from build123d import *

# Parameters (mm, degrees)
ESQUISSE1_W                                       = 50
ESQUISSE1_H                                       = 60
ESQUISSE1_R                                       = 14.5
BOSS_EXTRU_1_DEPTH                                = 10
ESQUISSE2_R                                       = 21.3
BOSS_EXTRU_2_DEPTH                                = 65.3
BOSS_EXTRU_3_START                                = -25
BOSS_EXTRU_3_DEPTH                                = 25
ENL_V_START                                       = 22
ENL_V_MAT_EXTRU_1_DEPTH                           = 22
CHAMBRAGE_POUR_VIS_SIX_PANS_CREUX_M41_D           = 4.5
CHAMBRAGE_POUR_VIS_SIX_PANS_CREUX_M41_CBORE_D     = 8
CHAMBRAGE_POUR_VIS_SIX_PANS_CREUX_M41_CBORE_DEPTH = 4.4
CHAMBRAGE_POUR_VIS_SIX_PANS_CREUX_M42_D           = 4.8
CHAMBRAGE_POUR_VIS_SIX_PANS_CREUX_M42_CBORE_D     = 8
CHAMBRAGE_POUR_VIS_SIX_PANS_CREUX_M42_CBORE_DEPTH = 4.4
BOSS_EXTRU_4_DEPTH                                = 30
CONG_1_R                                          = 4
CONG_2_R                                          = 4


with BuildPart() as part:
    # Esquisse1 → Boss.-Extru.1 (new body)
    with BuildSketch(Plane(origin=(0, 0, 0), x_dir=(1, 0, 0), z_dir=(0, 1, 0))):
        with Locations((25, 30)):
            Rectangle(ESQUISSE1_W, ESQUISSE1_H)
        with Locations(Location((25, 30, 0), (0, 0, 270))):
            Circle(ESQUISSE1_R, mode=Mode.SUBTRACT)
    extrude(amount=BOSS_EXTRU_1_DEPTH)

    # Esquisse2 → Boss.-Extru.2 (add)
    with BuildSketch(Plane(origin=(0, 10, 0), x_dir=(1, 0, 0), z_dir=(0, 1, 0))):
        with BuildLine():
            ThreePointArc((50, 41.456439237), (25, 57.5), (0, 41.456439237))
            Line((0, 41.456439237), (0, 18.543560763))
            ThreePointArc((0, 18.543560763), (25, 2.5), (50, 18.543560763))
            Line((50, 18.543560763), (50, 41.456439237))
        make_face()
        with Locations(Location((25, 30, 0), (0, 0, 270))):
            Circle(ESQUISSE2_R, mode=Mode.SUBTRACT)
    extrude(amount=BOSS_EXTRU_2_DEPTH)

    # Esquisse3 → Boss.-Extru.3 (add)
    with BuildSketch(Plane(origin=(0, 75.3, 0), x_dir=(1, 0, 0), z_dir=(0, 1, 0)).offset(BOSS_EXTRU_3_START)):
        with BuildLine():
            ThreePointArc((50, 18.543560763), (49.08967559, 16.735855475), (48.048861143, 15))
            Line((48.048861143, 15), (62.5, 15))
            Line((62.5, 15), (62.5, 45))
            Line((62.5, 45), (48.048861143, 45))
            ThreePointArc((48.048861143, 45), (49.08967559, 43.264144525), (50, 41.456439237))
            ThreePointArc((50, 41.456439237), (51.867731575, 35.8630197), (52.5, 30))
            ThreePointArc((52.5, 30), (51.867731575, 24.1369803), (50, 18.543560763))
        make_face()
        with BuildLine():
            Line((50, 41.456439237), (50, 18.543560763))
            ThreePointArc((50, 18.543560763), (51.867731575, 24.1369803), (52.5, 30))
            ThreePointArc((52.5, 30), (51.867731575, 35.8630197), (50, 41.456439237))
        make_face()
    extrude(amount=BOSS_EXTRU_3_DEPTH)

    # Esquisse4 → Enlèv. mat.-Extru.1 (cut)
    with BuildSketch(Plane(origin=(0, 75.3, -75.3), x_dir=(1, 0, 0), z_dir=(0, -1, 0)).offset(ENL_V_START)):
        with BuildLine():
            ThreePointArc((46.3, 45.3), (45.777219327, 40.609887311), (44.234539246, 36.15))
            Line((44.234539246, 36.15), (60, 36.15))
            Line((60, 36.15), (60, 54.45))
            Line((60, 54.45), (44.234539246, 54.45))
            ThreePointArc((44.234539246, 54.45), (45.777219327, 49.990112689), (46.3, 45.3))
        make_face()
    extrude(amount=-ENL_V_MAT_EXTRU_1_DEPTH, mode=Mode.SUBTRACT)

    # Chambrage pour vis à six pans creux M41 (through all)
    with Locations(Plane(origin=(5, 10, -55), x_dir=(0, 0, 1), z_dir=(0, 1, 0))):
        with Locations((0, 0), (0, 40), (50, 40), (50, 0)):
            CounterBoreHole(CHAMBRAGE_POUR_VIS_SIX_PANS_CREUX_M41_D / 2, CHAMBRAGE_POUR_VIS_SIX_PANS_CREUX_M41_CBORE_D / 2, CHAMBRAGE_POUR_VIS_SIX_PANS_CREUX_M41_CBORE_DEPTH)

    # Chambrage pour vis à six pans creux M42 (through all)
    with Locations(Plane(origin=(25, 0, -12.5), x_dir=(0, 0, -1), z_dir=(0, -1, 0))):
        with Locations((0, 0), (17.5, 17.5), (35, 0), (17.5, -17.5)):
            CounterBoreHole(CHAMBRAGE_POUR_VIS_SIX_PANS_CREUX_M42_D / 2, CHAMBRAGE_POUR_VIS_SIX_PANS_CREUX_M42_CBORE_D / 2, CHAMBRAGE_POUR_VIS_SIX_PANS_CREUX_M42_CBORE_DEPTH)

    # Esquisse11 → Boss.-Extru.4 (add)
    with BuildSketch(Plane.XY.offset(-15)):
        Polygon((48.048861143, 50.3), (48.048861143, 15.134837214), (62.5, 50.3), align=None)
    extrude(amount=-BOSS_EXTRU_4_DEPTH)

    # Congé1
    cong_1_edges = [part.edges().sort_by_distance(p)[0] for p in [
        (0, 5, -60),
        (50, 5, -60),
        (50, 5, 0),
        (0, 5, 0),
    ]]
    fillet(cong_1_edges, radius=CONG_1_R)

    # Congé2
    # the kernel refuses this fillet: 4 mm, written as the material it takes off along each edge
    with BuildSketch(Plane(origin=(58.5, 51.089853485, -41), x_dir=(1, 0, 0), z_dir=(0, 0, -1))) as cong_2_piece_1_section:
        Polygon((0, 0), (CONG_2_R, 0), (CONG_2_R, CONG_2_R * 0.197463371222), (CONG_2_R * 0.924943038794, CONG_2_R * 0.38010574185), align=None)
    cong_2_piece_1 = extrude(amount=CONG_2_R, mode=Mode.PRIVATE)
    cong_2_piece_1 = cong_2_piece_1 - Plane(origin=(58.5, 51.089853485, -41), x_dir=(-0.9810563283506197, 0.19372268995448388, 0), z_dir=(0, 0, -1)) * Sphere(CONG_2_R, mode=Mode.PRIVATE)
    add(cong_2_piece_1, mode=Mode.SUBTRACT)
    with BuildSketch(Plane(origin=(58.5, 51.089853485, -19), x_dir=(1, 0, 0), z_dir=(0, 0, 1))) as cong_2_piece_2_section:
        Polygon((0, 0), (CONG_2_R, 0), (CONG_2_R, -CONG_2_R * 0.197463371222), (CONG_2_R * 0.924943038794, -CONG_2_R * 0.38010574185), align=None)
    cong_2_piece_2 = extrude(amount=CONG_2_R, mode=Mode.PRIVATE)
    cong_2_piece_2 = cong_2_piece_2 - Plane(origin=(58.5, 51.089853485, -19), x_dir=(-0.9810563283506197, 0.19372268995448388, 0), z_dir=(0, 0, 1)) * Sphere(CONG_2_R, mode=Mode.PRIVATE)
    add(cong_2_piece_2, mode=Mode.SUBTRACT)
    with BuildSketch(Plane(origin=(62.5, 51.089853485, -45), x_dir=(-1, 0, 0), z_dir=(0, 1, 0))) as cong_2_piece_3:
        with BuildLine():
            CenterArc((CONG_2_R, CONG_2_R), CONG_2_R, 180, 90)
            Line((0, CONG_2_R), (0, 0))
            Line((0, 0), (CONG_2_R, 0))
        make_face()
    extrude(amount=34.210146515, mode=Mode.SUBTRACT)
    with BuildSketch(Plane(origin=(62.5, 50.3, -19), x_dir=(-0.3801057418499003, -0.9249430387935988, 0), z_dir=(0, 0, -1))) as cong_2_piece_4:
        with BuildLine():
            CenterArc((CONG_2_R * 0.197463371222, CONG_2_R), CONG_2_R, 247.659767296, 22.340232704)
            Line((-CONG_2_R * 0.182642370628, CONG_2_R * 0.0750569612064), (0, 0))
            Line((0, 0), (CONG_2_R * 0.197463371222, 0))
        make_face()
    extrude(amount=22, mode=Mode.SUBTRACT)
    with BuildSketch(Plane(origin=(62.5, 51.089853485, -15), x_dir=(-1, 0, 0), z_dir=(0, 1, 0))) as cong_2_piece_5:
        with BuildLine():
            CenterArc((CONG_2_R, -CONG_2_R), CONG_2_R, 90, 90)
            Line((0, -CONG_2_R), (0, 0))
            Line((0, 0), (CONG_2_R, 0))
        make_face()
    extrude(amount=34.210146515, mode=Mode.SUBTRACT)
    with BuildSketch(Plane(origin=(62.5, 75.3, -5), x_dir=(-1, 0, 0), z_dir=(0, 0, -1))) as cong_2_piece_6:
        with BuildLine():
            CenterArc((CONG_2_R, -CONG_2_R), CONG_2_R, 90, 90)
            Line((0, -CONG_2_R), (0, 0))
            Line((0, 0), (CONG_2_R, 0))
        make_face()
    extrude(amount=50, mode=Mode.SUBTRACT)
    with BuildSketch(Plane(origin=(44.247803725, 5.885406826, -45), x_dir=(0, 0, 1), z_dir=(0.38010574184990287, 0.9249430387935978, 0))) as cong_2_piece_7_section:
        with BuildLine():
            CenterArc((CONG_2_R, -CONG_2_R), CONG_2_R, 90, 90)
            Line((0, -CONG_2_R), (0, 0))
            Line((0, 0), (CONG_2_R, 0))
        make_face()
    cong_2_piece_7 = extrude(amount=47.228879898, mode=Mode.PRIVATE)
    cong_2_piece_7 = split(cong_2_piece_7, bisect_by=Plane(origin=(50, 20.820652224, -44.39379807), z_dir=(-1, 0, 0)), keep=Keep.TOP, mode=Mode.PRIVATE)
    cong_2_piece_7 = cong_2_piece_7 - Plane(origin=(25, 20.820652224, -30), x_dir=(0.909090909090922, 0, -0.4165977904505028), z_dir=(0, -1, 0)) * Cylinder(27.5, 111, mode=Mode.PRIVATE)
    add(cong_2_piece_7, mode=Mode.SUBTRACT)
    with BuildSketch(Plane(origin=(44.247803725, 5.885406826, -45), x_dir=(0, 0, 1), z_dir=(0.38010574184990287, 0.9249430387935978, 0))) as cong_2_piece_8_section:
        with BuildLine():
            CenterArc((CONG_2_R, -CONG_2_R), CONG_2_R, 90, 90)
            Line((0, -CONG_2_R), (0, 0))
            Line((0, 0), (CONG_2_R, 0))
        make_face()
    cong_2_piece_8 = extrude(amount=47.228879898, mode=Mode.PRIVATE)
    cong_2_piece_8 = split(cong_2_piece_8, bisect_by=Plane(origin=(50, 19.946502093, -41.15906608), z_dir=(1, 0, 0)), keep=Keep.TOP, mode=Mode.PRIVATE)
    cong_2_piece_8 = cong_2_piece_8 & Plane(origin=(25, 19.946502093, -30), x_dir=(0.909090909090922, 0, -0.4165977904505028), z_dir=(0, -1, 0)) * Cylinder(27.5, 111, mode=Mode.PRIVATE)
    add(cong_2_piece_8, mode=Mode.SUBTRACT)
    with BuildSketch(Plane(origin=(44.247803725, 5.885406826, -45), x_dir=(0, 0, 1), z_dir=(0.38010574184990287, 0.9249430387935978, 0))) as cong_2_piece_9_section:
        with BuildLine():
            CenterArc((CONG_2_R, -CONG_2_R), CONG_2_R, 90, 90)
            Line((0, -CONG_2_R), (0, 0))
            Line((0, 0), (CONG_2_R, 0))
        make_face()
    cong_2_piece_9 = extrude(amount=47.228879898, mode=Mode.PRIVATE)
    cong_2_piece_9 = split(cong_2_piece_9, bisect_by=Plane(origin=(50, 35.999636331, -44.058905406), z_dir=(1, 0, 0)), keep=Keep.TOP, mode=Mode.PRIVATE)
    cong_2_piece_9 = cong_2_piece_9 - Plane(origin=(25, 35.999636331, -30), x_dir=(0.909090909090922, 0, -0.4165977904505028), z_dir=(0, -1, 0)) * Cylinder(27.5, 111, mode=Mode.PRIVATE)
    add(cong_2_piece_9, mode=Mode.SUBTRACT)
    with BuildSketch(Plane(origin=(44.247803725, 5.885406826, -15), x_dir=(0, 0, -1), z_dir=(0.38010574184990287, 0.9249430387935978, 0))) as cong_2_piece_10_section:
        with BuildLine():
            CenterArc((CONG_2_R, CONG_2_R), CONG_2_R, 180, 90)
            Line((0, CONG_2_R), (0, 0))
            Line((0, 0), (CONG_2_R, 0))
        make_face()
    cong_2_piece_10 = extrude(amount=47.228879898, mode=Mode.PRIVATE)
    cong_2_piece_10 = split(cong_2_piece_10, bisect_by=Plane(origin=(50, 20.820650569, -15.60620042), z_dir=(-1, 0, 0)), keep=Keep.TOP, mode=Mode.PRIVATE)
    cong_2_piece_10 = cong_2_piece_10 - Plane(origin=(25, 20.820650569, -30), x_dir=(-0.9090909090909031, 0, 0.4165977904505442), z_dir=(0, -1, 0)) * Cylinder(27.5, 111, mode=Mode.PRIVATE)
    add(cong_2_piece_10, mode=Mode.SUBTRACT)
    with BuildSketch(Plane(origin=(44.247803725, 5.885406826, -15), x_dir=(0, 0, -1), z_dir=(0.38010574184990287, 0.9249430387935978, 0))) as cong_2_piece_11_section:
        with BuildLine():
            CenterArc((CONG_2_R, CONG_2_R), CONG_2_R, 180, 90)
            Line((0, CONG_2_R), (0, 0))
            Line((0, 0), (CONG_2_R, 0))
        make_face()
    cong_2_piece_11 = extrude(amount=47.228879898, mode=Mode.PRIVATE)
    cong_2_piece_11 = split(cong_2_piece_11, bisect_by=Plane(origin=(50, 19.946502096, -18.840933919), z_dir=(1, 0, 0)), keep=Keep.TOP, mode=Mode.PRIVATE)
    cong_2_piece_11 = cong_2_piece_11 & Plane(origin=(25, 19.946502096, -30), x_dir=(-0.9090909090909031, 0, 0.4165977904505442), z_dir=(0, -1, 0)) * Cylinder(27.5, 111, mode=Mode.PRIVATE)
    add(cong_2_piece_11, mode=Mode.SUBTRACT)
    with BuildSketch(Plane(origin=(44.247803725, 5.885406826, -15), x_dir=(0, 0, -1), z_dir=(0.38010574184990287, 0.9249430387935978, 0))) as cong_2_piece_12_section:
        with BuildLine():
            CenterArc((CONG_2_R, CONG_2_R), CONG_2_R, 180, 90)
            Line((0, CONG_2_R), (0, 0))
            Line((0, 0), (CONG_2_R, 0))
        make_face()
    cong_2_piece_12 = extrude(amount=47.228879898, mode=Mode.PRIVATE)
    cong_2_piece_12 = split(cong_2_piece_12, bisect_by=Plane(origin=(50, 35.999636337, -15.941094594), z_dir=(1, 0, 0)), keep=Keep.TOP, mode=Mode.PRIVATE)
    cong_2_piece_12 = cong_2_piece_12 - Plane(origin=(25, 35.999636337, -30), x_dir=(-0.9090909090909031, 0, 0.4165977904505442), z_dir=(0, -1, 0)) * Cylinder(27.5, 111, mode=Mode.PRIVATE)
    add(cong_2_piece_12, mode=Mode.SUBTRACT)


solid = part.part
Geometry: final body of the model. Coordinates: model frame, mm. A direction names the side the tool comes from. Round coordinates to 2 decimals unless told otherwise and drop trailing zeros. Loops run counter-clockwise (first coordinate to the right, second up) from the corner with the lowest first, then second, coordinate; pieces in that order, holes last. Notation, with made-up numbers: (10, 79) -> (52, 79) arc R9 cw to (52, 89) -> close; hole circle Ø6 at (20.5, -0.5). An arc over 180 degrees is marked (long way). One line per question, with ' | ' between items. Start each with the question number.
1. Set-up query: faces 5 (the face through (46.5, 2.2, -30.1)), 6 (the face through (3, 5.6, -53)), 7 (the face through (61.359, 63.025, -43.797)). Return all of +Z, -Z, +X, -X, +Y, -Y with unobstructed straight access to the full face (end or side cutting, diameter ignored); none if empty.
2. Section A-A on y = 64.5. Output: boundary loops of the cut face in (x, z).
3. Mould query, pull axis Z, two halves, no side actions, for faces 1 (the face through (54.82, 34.62, -43.8)), 2 (the face through (22.657, 7.239, -13.02)), 3 (the face through (61.297, 63.025, -16.141)), 4 (the face through (62.5, 61, -30)). Classes: pulls with the +Z half, pulls with the -Z half, needs draft (parallel to the pull), parting line crosses it, or undercut.
4. Section D-D on z = -12.5. Output: boundary loops of the cut face in (x, y), and give its area (3 significant figures).
5. Section C-C on x = 37.5. Output: boundary loops of the cut face in (y, z), and give its area (3 significant figures).
6. Line query: line 1 along X through (y, z) = (7, -30); line 2 along Z through (x, y) = (25, 27.5); line 3 along X through (y, z) = (8, -5). Output: solid intervals per line, ascending. Write a range as [from, to].
7. Section B-B on z = -30. Count the separate pieces of the cut face and the enclosed holes in it, and give its area (3 significant figures).
8. Contact query for flat-ended pins moving along their axis: pin 1 (4 mm diameter, centred on x = 35.5, y = 27.5, fed in from +Z); pin 2 (10 mm diameter, centred on x = 45.5, y = 48, fed in from -Z); pin 3 (6 mm diameter, centred on x = 7.5, z = -30.5, fed in from -Y); pin 4 (6 mm diameter, centred on x = 26, z = -48, fed in from -Y). Output: stop coordinate, or through.
Returned:
1) face 5: -Y | face 6: +Y | face 7: -Z, +X, +Y, -Y
2) outline: (0, -41.46) arc R27.5 ccw to (48.05, -45) -> (58.5, -45) arc R4 ccw to (62.5, -41) -> (62.5, -19) arc R4 ccw to (58.5, -15) -> (48.05, -15) arc R27.5 ccw to (0, -18.54) -> close; hole (44.23, -39.15) -> (60, -39.15) -> (60, -20.85) -> (44.23, -20.85) arc R21.3 ccw (long way) to start
3) face 1: pulls with the -Z half | face 2: undercut | face 3: pulls with the +Z half | face 4: needs draft
4) outline: (0, 0) -> (21, 0) -> (21, 4.4) -> (22.6, 4.4) -> (22.6, 10) -> (12.86, 10) -> (12.86, 75.3) -> (3.79, 75.3) -> (3.79, 10) -> (0, 10) -> close; (27.4, 4.4) -> (29, 4.4) -> (29, 0) -> (50, 0) -> (50, 10) -> (46.21, 10) -> (46.21, 75.3) -> (37.14, 75.3) -> (37.14, 10) -> (27.4, 10) -> close | area: 1,620 mm2
5) outline: (0, -60) -> (10, -60) -> (10, -54.49) -> (75.3, -54.49) -> (75.3, -47.25) -> (10, -47.25) -> (10, -37.35) -> (0, -37.35) -> close; (0, -22.65) -> (10, -22.65) -> (10, -12.75) -> (75.3, -12.75) -> (75.3, -5.51) -> (10, -5.51) -> (10, 0) -> (0, 0) -> close | area: 1,400 mm2
6) line 1: x = [0, 5.1], [9.9, 10.5], [39.5, 40.1], [44.9, 50] | line 2: z = [-57.5, -51.3], [-8.7, -2.5] | line 3: x = [0, 1], [9, 41], [49, 50]
7) separate pieces: 4 | enclosed holes: 0 | area: 776 mm2
8) pin 1: stops at z = -3.85 | pin 2: stops at z = -52.72 | pin 3: stops at y = 4.4 | pin 4: stops at y = 0
